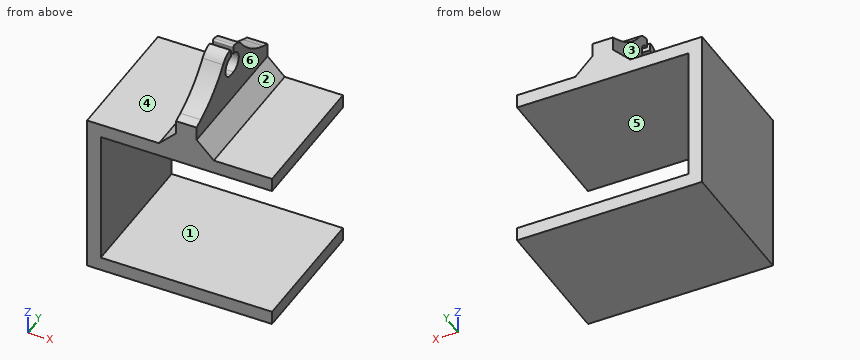
Autodesk Fusion 360 part; units mm, degrees
sketch "Sketch1" plane through (0, 0, 0) normal (0, 0, 1) x (1, 0, 0)
  line L0 (-12.5, 10) -> (12.5, 10)
  line L1 (12.5, 10) -> (12.5, -10)
  line L2 (12.5, -10) -> (-12.5, -10)
  line L3 (-12.5, -10) -> (-12.5, 10)
  dimension "d1" = 25
  dimension "d2" = 12.5
  dimension "d3" = 20
  dimension "d4" = 10
extrude "Extrude1" add sketch "Sketch1" along normal blind 2
sketch "Sketch2" plane through (0, 0, 2) normal (0, 0, 1) x (-1, 0, 0)
  line L0 (12.5, 10) -> (-12.5, 10)
  line L1 (-12.5, 10) -> (-12.5, -10)
  line L2 (-12.5, -10) -> (12.5, -10)
  line L3 (12.5, -10) -> (12.5, 10)
  line L4 (12.5, 10) -> (14.5, 10)
  line L5 (14.5, 10) -> (14.5, -10)
  line L6 (14.5, -10) -> (12.5, -10)
  line L7 (12.5, -10) -> (12.5, 10)
  dimension "d7" = 2
extrude "Extrude2" add sketch "Sketch2" along normal blind -2 and the other way blind -20 contours L3 L4 L5 L6 L7
sketch "Sketch3" plane through (0, 0, 22) normal (0, 0, 1) x (-1, 0, 0)
  line L0 (12.5, -10) -> (14.5, -10)
  line L1 (14.5, -10) -> (14.5, 10)
  line L2 (14.5, 10) -> (12.5, 10)
  line L3 (12.5, 10) -> (12.5, -10)
  line L4 (14.5, -10) -> (-12.5, -10)
  line L5 (-12.5, -10) -> (-12.5, 10)
  line L6 (-12.5, 10) -> (14.5, 10)
  line L7 (14.5, 10) -> (14.5, -10)
  point P0 (-12.5, 10)
  dimension "d12" = 27
extrude "Extrude3" add sketch "Sketch3" along normal blind 2
ref_plane "WorkPlane1" through (0, 0, 23) normal (1, 0, 0) x (0, 1, 0)
sketch "Sketch8" plane through (0, 0, 0) normal (1, 0, 0) x (0, 1, 0)
  line L0 (-0.375, 37.553) -> (0.375, 37.553)
  line L1 (-9.7103, 24) -> (10, 24)
  circle A0 centre (-0.375, 32) radius 2.75
  circle A1 centre (0.375, 32) radius 2.75
  line L2 (0.375, 37.553) -> (0.375, 32)
  circle A2 centre (0.375, 32) radius 1.5
  line L3 (0.375, 32) -> (0.375, 24)
  circle A3 centre (-0.375, 32) radius 1.5
  line L4 (-0.375, 32) -> (-0.375, 24)
  line L5 (-0.375, 32) -> (-0.375, 37.553)
  line L6 (10, 24) -> (-10, 24)
  line L7 (-10, 24) -> (-10, 28.5)
  line L8 (-10, 28.5) -> (10, 28.5)
  line L9 (10, 28.5) -> (10, 24)
  line L10 (-5, 30.5) -> (5, 30.5)
  line L11 (-10, 28.5) -> (-5, 30.5)
  line L12 (5, 30.5) -> (10, 28.5)
  point P0 (-9.7103, 23.053)
  point P1 (0, 22)
  point P2 (10, 23.053)
  point P3 (10, 24)
  point P4 (-10, 24)
  dimension "d73" = 5.5
  dimension "d74" = 5.5
  dimension "d75" = 10
  dimension "d76" = 0.75
  dimension "d77" = 0.375
  dimension "d78" = 3
  dimension "d79" = 3
  dimension "d80" = 2
  dimension "d93" = 3.5
  dimension "d101" = 1.5
  dimension "d102" = 10
  dimension "d103" = 5
extrude "Extrude11" add 1 faces at (-4.1667, 3.3333, 2) along direction (0, 0, 1) blind 0.25
extrude "Extrude12" cut 1 faces at (-5.5, -3.3333, 0) along direction (0, 0, 1) blind 0.25
extrude "Extrude14" add sketch "Sketch8" along normal mid plane 3 contours A0 A1 L5 L10 | A0 A1 L2 L10 | A0 A1 L4 L10 | A0 L4 L8 L10 L11 | A1 A3 L5 L10 | A0 L2 A2 L10 | A0 A1 L4 | A0 A1 L3 L4 L8 | A1 L4 L10 | A1 L3 L8 L10 L12 | A0 A1 L3 L10 | A0 A1 L3 L4 L10 | A0 A1 L3 | L1 L3 L4 L6 L8 | L1 L4 L6 L7 L8 | A0 L3 L10 | L1 L3 L6 L8 L9
chamfer "Chamfer2" distance 2.5 angle 45 2 edges at (1.5, 0, 24) (-1.5, 0, 24)
fillet "Fillet16" radius 15 2 edges at (0, -2.6799, 30.5) (0, 2.6799, 30.5)
fillet "Fillet16" radius 0.25 2 edges at (0, 0.375, 34.75) (0, -0.375, 34.75)
fillet "Fillet16" radius 2 2 edges at (0, -5, 30.5) (0, 5, 30.5)
equation "d77 = ( 0.75 / 2 ) * 1 mm"
Design review of the part built by this model. Coordinates are the model's own, in mm. Face numbers are marked on the shaded views. A direction names the side the tool comes from. Coordinates: 2 decimals unless noted, no trailing zeros. Write each loop counter-clockwise with the first axis right and the second up, starting at its lowest first coordinate (ties: lowest second). Pieces come first, ordered by that corner, then holes. Notation, with made-up numbers: (-9, 7.5) -> (41, 7.5) arc R14 cw to (41, 23.5) -> close; hole circle Ø6 at (57, -36.5). An arc over 180 degrees is marked (long way). Write each question's results on one line, items separated by ' | '. Start each with the question number.
(1) Take a section at B-B on x = 3.25. Write out the cut boundary in (y, z), and give its area (3 significant figures).
(2) Take a section at C-C on z = 21. Write out the cut boundary in (x, y), and give its area (3 significant figures).
(3) For line 1 along Z through (x, y) = (11, -5.5); line 2 along X through (y, z) = (-6, 6); line 3 along Z through (x, y) = (2.5, 1), list the stretches that pass through material, from the lowest coordinate up. Write a range as from..to.
(4) Clearance check with flat-ended pins moving along their axes: P1, Ø9.5, axis at x = 10, y = -4.5, coming from the +Z side; P2, Ø12, axis at x = 4, z = 5, coming from the -Y side; P3, Ø0.6, axis at x = 0, y = 0, coming from the +Z side; P4, Ø8, axis at x = 1, z = 9.5, coming from the -Y side. State where each tip first meets the part, or that it passes through.
(5) Take a section at A-A on x = -3. Write out the cut boundary in (y, z), and give its area (3 significant figures).
(6) Tool access review of the marked faces 4, 5 and 6: name each direction out of +Z, -Z, +X, -X, +Y, -Y from which nothing blocks a thin tool from reaching the whole face with its end or side.
(7) The part is to be moulded in two halves that separate along Z. For the marked faces 1, 2 and 3, say which applies: pulls with the +Z half, pulls with the -Z half, needs draft (parallel to the pull), parting line crosses it, or undercut.
Results found:
1) outline: (-10, 0.25) -> (10, 0.25) -> (10, 2.25) -> (-10, 2.25) -> close; (-10, 22) -> (10, 22) -> (10, 24.75) -> (-10, 24.75) -> close | area: 95.0 mm2
2) outline: (-14.5, -10) -> (-12.5, -10) -> (-12.5, 10) -> (-14.5, 10) -> close | area: 40.0 mm2
3) line 1: z = 0.25..2.25, 22..24 | line 2: x = -14.5..-12.5 | line 3: z = 0.25..2.25, 22..25.5
4) P1: stops at z = 24 | P2: stops at y = -10 | P3: stops at z = 30.5 | P4: passes through
5) outline: (-10, 0.25) -> (10, 0.25) -> (10, 2.25) -> (-10, 2.25) -> close; (-10, 22) -> (10, 22) -> (10, 25) -> (-10, 25) -> close | area: 100 mm2
6) face 4: +Z, -X, +Y, -Y | face 5: +X, +Y, -Y | face 6: +Z, +X, +Y, -Y
7) face 1: undercut | face 2: pulls with the +Z half | face 3: needs draft
